Study the drawing (mm; zero at the part's minimum x, y, z) and answer. Round coordinates to 2 decimals unless told otherwise and drop trailing zeros. Write each loop counter-clockwise with the first axis right and the second up, starting at its lowest first coordinate (ties: lowest second). Pieces come first, ordered by that corner, then holes. Notation, with made-up numbers: (50, -2) - (62, -2) arc R16 ccw to (62, 13) - close; hole circle Ø3 at (65.5, 67.5). An arc over 180 degrees is marked (long way). Use one line per item in the form item = value. Start each with the question number.
1) The part is cut by section B-B, the plane y = 0.25. Give the vertices of the cut face in (x, z).
2) For a pull along Z with two mould halves and no side action, classify the marked faces 1, 2 and 3 as released by +Z, released by -Z, zero draft, split by the parting line, or undercut.
3) Consider line 1 along Z through (x, y) = (1, 0.6); line 2 along X through (y, z) = (1.25, 7.75); line 3 along Z through (x, y) = (0.45, 0.9) (1 decimal). Determine where each line is inside the solid, lowest interval first. Write a range as from..to.
4) The part is cut by section C-C, the plane y = 1.45. Give the vertices of the cut face in (x, z).
5) The part is cut by section A-A, the plane x = 1. Give the vertices of the cut face in (y, z).
6) The part is cut by section D-D, the plane z = 2.25. Give the vertices of the cut face in (x, y).
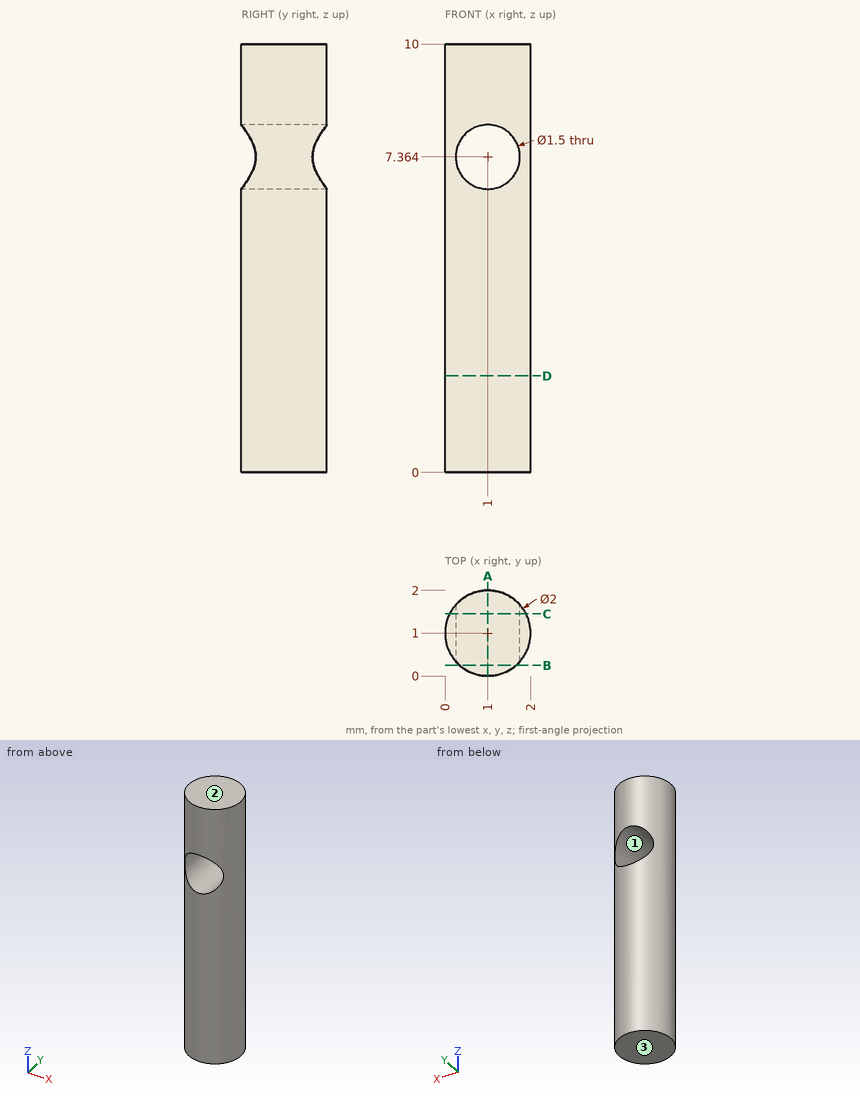
Geometry results:
q1.outline = (0.34, 0) - (1.66, 0) - (1.66, 7.01) arc R0.75 cw to (0.34, 7.01) - close; (0.34, 7.72) arc R0.75 cw to (1.66, 7.72) - (1.66, 10) - (0.34, 10) - close
q2.face_1 = undercut
q2.face_2 = released by +Z
q2.face_3 = released by -Z
q3.line_1 = 0..6.61, 8.11..10
q3.line_2 = 0.03..0.36, 1.64..1.97
q3.line_3 = 0..6.9, 7.9..10
q4.outline = (0.11, 0) - (1.89, 0) - (1.89, 10) - (0.11, 10) - close; hole circle Ø1.5 at (1, 7.36)
q5.outline = (0, 0) - (2, 0) - (2, 6.61) - (0, 6.61) - close; (0, 8.11) - (2, 8.11) - (2, 10) - (0, 10) - close
q6.outline = circle Ø2 at (1, 1)
